Design review of the part built by this model. Coordinates are the model's own, in mm. A direction names the side the tool comes from. Coordinates: 2 decimals unless noted, no trailing zeros. Loops run counter-clockwise (first coordinate to the right, second up) from the corner with the lowest first, then second, coordinate; pieces in that order, holes last. Notation, with made-up numbers: (-40, -34) - (-24, -34) arc R11 ccw to (-24, -13) - close; hole circle Ø7 at (86, 35). An arc over 180 degrees is marked (long way). Use one line per item in the form item = value. Start each with the question number.
(1) Tool access review of faces 1 (the face through (0, 4, -12)), 2 (the face through (0, -9, 4)), 3 (the face through (0, 0, 20)): name each direction out of +Z, -Z, +X, -X, +Y, -Y from which nothing blocks a thin tool from reaching the whole face with its end or side.
(2) Add section C-C (x = 9.5). State the section outline as (y, z) points.
(3) The part is to be moulded in two halves that separate along Y. For faces 4 (the face through (11.69, 0.12, 1.08)), 5 (the face through (0, 15, 5)), 6 (the face through (-2, 5, 0)), 7 (the face through (13, -12, 4)), say which applies: pulls with the +Y half, pulls with the -Y half, needs draft (parallel to the pull), parting line crosses it, or undercut.
(4) Clearance check with flat-ended pins moving along their axes: pin 1 Ø11.5 at (y, z) = (5, 0) entering from +X; pin 2 Ø8 at (x, z) = (-4, 8.5) entering from -Y; pin 3 Ø1 at (x, y) = (-7, -9) entering from -Z. State where each tip first meets the part, or that it passes through.
(5) Add section B-B (y = 5). State the section outline as (x, z) points, plus the area to 3 significant figures.
(6) For L1, parallel to Y at x = 6, z = 0; L2, parallel to X at y = -1.75, z = -16; L3, parallel to X at y = -13.5, z = 17, list the stretches that pass through material, from the lowest coordinate up.
(7) Add section D-D (z = -3). State the section outline as (x, y) points.
(8) Add section A-A (z = -17). State the section outline as (x, y) points, plus the area to 3 significant figures.
```python
from build123d import *

# Parameters (mm, degrees)
SKETCH_1_W               = 50
SKETCH_1_H               = 30
EXTRUDE_1_DEPTH          = 20
CUT_EXTRUDE_2_DEPTH      = 36.355339059
CUT_EXTRUDE_2_DEPTH_BACK = 36.355339059
SKETCH_2_W               = 26
SKETCH_2_H               = 6
SKETCH_4_W               = 38
SKETCH_4_H               = 8
CUT_EXTRUDE_3_DEPTH      = 44.874821937
SKETCH_5_R               = 5
CUT_EXTRUDE_5_DEPTH      = 27


with BuildPart() as part:
    # 草圖1 → 填料-伸長1 (new, symmetric)
    with BuildSketch(Plane.XY):
        Rectangle(SKETCH_1_W, SKETCH_1_H)
    extrude(amount=EXTRUDE_1_DEPTH, both=True)

    # 草圖2 → 除料-伸長2 (cut, two sides: drawn at the far end of the back side and taken through both)
    with BuildSketch(Plane.XY.offset(-CUT_EXTRUDE_2_DEPTH_BACK)):
        with Locations((0, -12)):
            Rectangle(SKETCH_2_W, SKETCH_2_H)
    extrude(amount=CUT_EXTRUDE_2_DEPTH + CUT_EXTRUDE_2_DEPTH_BACK, mode=Mode.SUBTRACT)

    # 草圖4 → 除料-伸長3 (cut, through all)
    with BuildSketch(Plane(origin=(0, 15, 0), x_dir=(1, 0, 0), z_dir=(0, 1, 0))):
        with Locations((0, 16)):
            Rectangle(SKETCH_4_W, SKETCH_4_H)
    extrude(amount=-CUT_EXTRUDE_3_DEPTH, mode=Mode.SUBTRACT)

    # 草圖5 → 除料-伸長5 (cut)
    with BuildSketch(Plane(origin=(25, 0, 0), x_dir=(0, 0, -1), z_dir=(1, 0, 0))):
        with Locations((0, 5)):
            Circle(SKETCH_5_R)
    extrude(amount=-CUT_EXTRUDE_5_DEPTH, mode=Mode.SUBTRACT)


solid = part.part
```
Computed values:
q1.face_1 = -Z, +Y, -Y
q1.face_2 = +Z, -Z, -Y
q1.face_3 = +Z, +X, -X, +Y, -Y
q2.outline = (-9, -12) - (15, -12) - (15, 20) - (-9, 20) - close; hole circle Ø10 at (5, 0)
q3.face_4 = undercut
q3.face_5 = pulls with the +Y half
q3.face_6 = undercut
q3.face_7 = needs draft
q4.pin_1 = 25
q4.pin_2 = -9
q4.pin_3 = -12
q5.outline = (-25, -20) - (-19, -20) - (-19, -12) - (19, -12) - (19, -20) - (25, -20) - (25, -5) - (-2, -5) - (-2, 5) - (25, 5) - (25, 20) - (-25, 20) - close
q5.area = 1,430 mm^2
q6.L1 = -9 to 0, 10 to 15
q6.L2 = -25 to -19, 19 to 25
q6.L3 = -25 to -13, 13 to 25
q7.outline = (-25, -15) - (-13, -15) - (-13, -9) - (13, -9) - (13, -15) - (25, -15) - (25, 1) - (-2, 1) - (-2, 9) - (25, 9) - (25, 15) - (-25, 15) - close
q8.outline = (-25, -15) - (-19, -15) - (-19, 15) - (-25, 15) - close; (19, -15) - (25, -15) - (25, 15) - (19, 15) - close
q8.area = 360 mm^2
